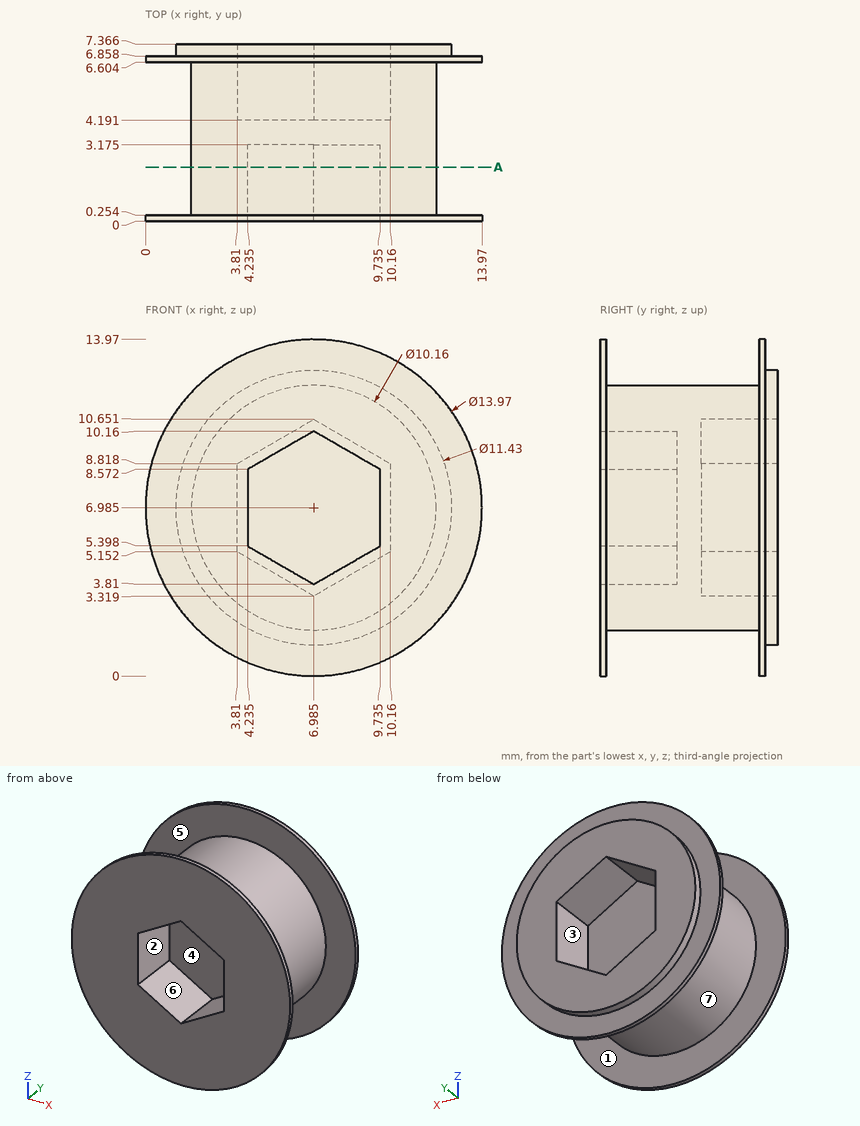
Here's the drawing with two shaded views (mm, measured from the low corner). I have some questions. A direction names the side the tool comes from. Coordinates: 2 decimals unless noted, no trailing zeros. Order: outer loops, then holes, each group sorted by start corner. A loop starts at its lowest first (then second) coordinate and runs counter-clockwise, first axis right, second up. Notation, with made-up numbers: (44, -27.5) -> (96, -27.5) arc R24 ccw to (96, 0.5) -> close; hole circle Ø2 at (70, -16). An arc over 180 degrees is marked (long way). One line per question, with ' | ' between items.
Q1. On a 3-axis mill with a long thin cutter (end or side, diameter ignored), from which of +Z, -Z, +X, -X, +Y, -Y can I reach the whole of each face in a straight line? I mean the marked faces 1, 2 and 3. Say none if no direction works.
Return value:
face 1: none | face 2: -Y | face 3: +Y
Q2. Thinking about a two-plate mould opening in Z: for the marked faces 4, 5, 6 and 7, which applies, pulls with the +Z half, pulls with the -Z half, needs draft (parallel to the pull), parting line crosses it, or undercut?
Return value:
face 4: undercut | face 5: needs draft | face 6: undercut | face 7: parting line crosses it
Q3. I'm going to push flat-ended pins straight in: P1, Ø1.6, axis at y = 5.5, z = 7, coming from the -X side (1 decimal); P2, Ø1.5, axis at x = 7.5, y = 5, coming from the +Z side (1 decimal); P3, Ø2, axis at x = 8, y = 5.5, coming from the -Z side (1 decimal). Where does each tip first touch, or does it pass through?
Return value:
P1: x = 1.9 | P2: z = 12.1 | P3: z = 1.9
Q4. Imagine slicing it at A-A on y = 2.25. Please give me the cut outline in (x, z) (1 decimal).
Return value:
outline: circle Ø10.2 at (7, 7); hole (4.2, 5.4) -> (7, 3.8) -> (9.7, 5.4) -> (9.7, 8.6) -> (7, 10.2) -> (4.2, 8.6) -> close
Q5. If I drill on L1, parallel to Y at x = 1.5, z = 7 (1 decimal); L2, parallel to Y at x = 4.5, z = 7.5 (1 decimal); L3, parallel to Y at x = 8.75, z = 9.5, over which ranges is the centre line in solid material (lowest first)?
Return value:
L1: 0 to 0.3, 6.6 to 7.4 | L2: 3.2 to 4.2 | L3: 0 to 4.19
